The model under review builds one solid part; all positions refer to its coordinate system, in mm. A direction names the side the tool comes from. Round coordinates to 2 decimals unless told otherwise and drop trailing zeros. Order: outer loops, then holes, each group sorted by start corner. A loop starts at its lowest first (then second) coordinate and runs counter-clockwise, first axis right, second up.
1) Consider section D-D (z = 20). Give the boundary of the cut face in (x, y) (3 decimals).
2) Mouldability with a two-part tool opening along X and no side actions: class faces 1 (the face through (3.175, 13, 13)), 2 (the face through (25, 23, 0)), 3 (the face through (8.389, 23.835, 10.494)), 4 (the face through (50.8, 13, 13)) as pulls with the +X half, pulls with the -X half, needs draft (parallel to the pull), parting line crosses it, or undercut.
3) Consider section B-B (z = 12.7). Give the boundary of the cut face in (x, y) (3 decimals).
4) Machinability: for faces 5 (the face through (37.599, 1.61, 10.494)), 6 (the face through (47.625, 13, 13)), which of the approach directions +Z, -Z, +X, -X, +Y, -Y give a long, thin tool a straight path to every point of the face, cutting with its end or side? Answer none if there is none.
5) Consider section C-C (x = 45.5). Give the boundary of the cut face in (y, z) (3 decimals).
6) To check wall thickness, follow L1, parallel to X at y = 23.9, z = 12.7; L2, parallel to Y at x = 44.5, z = 11.5 (3 decimals); L3, parallel to X at y = 21.5, z = 19 (3 decimals). State the ranges of each line that lie inside material, in increasing order.
7) Consider section A-A (y = 6.5). Give the boundary of the cut face in (x, z) (3 decimals), then the cut area to 3 significant figures.
from build123d import *

# Parameters (mm, degrees)
SKETCH1_W               = 50.8
SKETCH1_H               = 25.4
SKETCH1_W_2             = 44.45
SKETCH1_H_2             = 19.05
BOSS_EXTRUDE1_DEPTH     = 25.4
SKETCH8_R               = 3.2639
CUT_EXTRUDE1_DEPTH      = 1
CUT_EXTRUDE1_DEPTH_BACK = 26.4


with BuildPart() as part:
    # Sketch1 → Boss-Extrude1 (new body)
    with BuildSketch(Plane.XY):
        with Locations((25.4, 12.7)):
            Rectangle(SKETCH1_W, SKETCH1_H)
        with Locations((25.4, 12.7)):
            Rectangle(SKETCH1_W_2, SKETCH1_H_2, mode=Mode.SUBTRACT)
    extrude(amount=BOSS_EXTRUDE1_DEPTH)

    # Sketch8 → Cut-Extrude1 (cut, two sides)
    with BuildSketch(Plane(origin=(0, 25.4, 0), x_dir=(1, 0, 0), z_dir=(0, 1, 0))) as cut_extrude1_sk:
        with Locations((10.795, -12.7)):
            Circle(SKETCH8_R)
        with Locations((40.005, -12.7)):
            Circle(SKETCH8_R)
    extrude(amount=CUT_EXTRUDE1_DEPTH, mode=Mode.SUBTRACT)
    extrude(cut_extrude1_sk.sketch, amount=-CUT_EXTRUDE1_DEPTH_BACK, mode=Mode.SUBTRACT)


solid = part.part
Answer below:
1. outline: (0, 0) - (50.8, 0) - (50.8, 25.4) - (0, 25.4) - close; hole (3.175, 3.175) - (47.625, 3.175) - (47.625, 22.225) - (3.175, 22.225) - close
2. face 1: undercut
2. face 2: needs draft
2. face 3: undercut
2. face 4: pulls with the +X half
3. outline: (0, 0) - (7.531, 0) - (7.531, 3.175) - (3.175, 3.175) - (3.175, 22.225) - (7.531, 22.225) - (7.531, 25.4) - (0, 25.4) - close; (14.059, 0) - (36.741, 0) - (36.741, 3.175) - (14.059, 3.175) - close; (14.059, 22.225) - (36.741, 22.225) - (36.741, 25.4) - (14.059, 25.4) - close; (43.269, 0) - (50.8, 0) - (50.8, 25.4) - (43.269, 25.4) - (43.269, 22.225) - (47.625, 22.225) - (47.625, 3.175) - (43.269, 3.175) - close
4. face 5: +Y, -Y
4. face 6: +Z, -Z
5. outline: (0, 0) - (3.175, 0) - (3.175, 25.4) - (0, 25.4) - close; (22.225, 0) - (25.4, 0) - (25.4, 25.4) - (22.225, 25.4) - close
6. L1: x = 0 to 7.53, 14.06 to 36.74, 43.27 to 50.8
6. L2: y = 0 to 3.175, 22.225 to 25.4
6. L3: x = 0 to 3.175, 47.625 to 50.8
7. outline: (0, 0) - (3.175, 0) - (3.175, 25.4) - (0, 25.4) - close; (47.625, 0) - (50.8, 0) - (50.8, 25.4) - (47.625, 25.4) - close
7. area: 161 mm2
